Input: dimensioned drawing with shaded views. Units: mm. Origin: part minimum x, y, z. A direction names the side the tool comes from. Round coordinates to 2 decimals unless told otherwise and drop trailing zeros. Order: outer loops, then holes, each group sorted by start corner. A loop starts at its lowest first (then second) coordinate and runs counter-clockwise, first axis right, second up. Notation, with made-up numbers: (42.25, 47.5) - (62.25, 47.5) arc R13 cw to (62.25, 55.5) - close; hole circle Ø11 at (-16.75, 67). An arc over 180 degrees is marked (long way). Put each result on its own line as item: value. Start each with the question number.
(1) Pull-direction query (Y, two-part tool) for the marked faces 4, 5 and 6; classes: released by +Y, released by -Y, zero draft, split by the parting line, or undercut.
(2) Section B-B (x = 36). Output: boundary loops of the cut face in (y, z).
(3) Section D-D (z = 25.5). Output: boundary loops of the cut face in (x, y).
(4) Section C-C (y = 10). Output: boundary loops of the cut face in (x, z).
(5) Material intervals for L1, parallel to X at y = 60.5, z = 17.5; L2, parallel to Y at x = 11, z = 10; L3, parallel to Y at x = 30, z = 16, sorted ascending. Write a range as [from, to].
(6) Pin query (flat end, axial travel): P1, Ø6, axis at y = 64, z = 24, coming from the -X side; P2, Ø8, axis at y = 41, z = 14, coming from the -X side; P3, Ø20.5, axis at x = 13.5, y = 67, coming from the +Z side; P4, Ø1, axis at x = 31.5, y = 64, coming from the -Z side. Return the tip coordinate at first contact, or that it passes through.
(7) Access query for the marked faces 1, 2 and 3. Directions: +Z, -Z, +X, -X, +Y, -Y. A direction counts if a zero-diameter tool reaches every point of the face in a straight line with its end or side. Return the directions, or none.
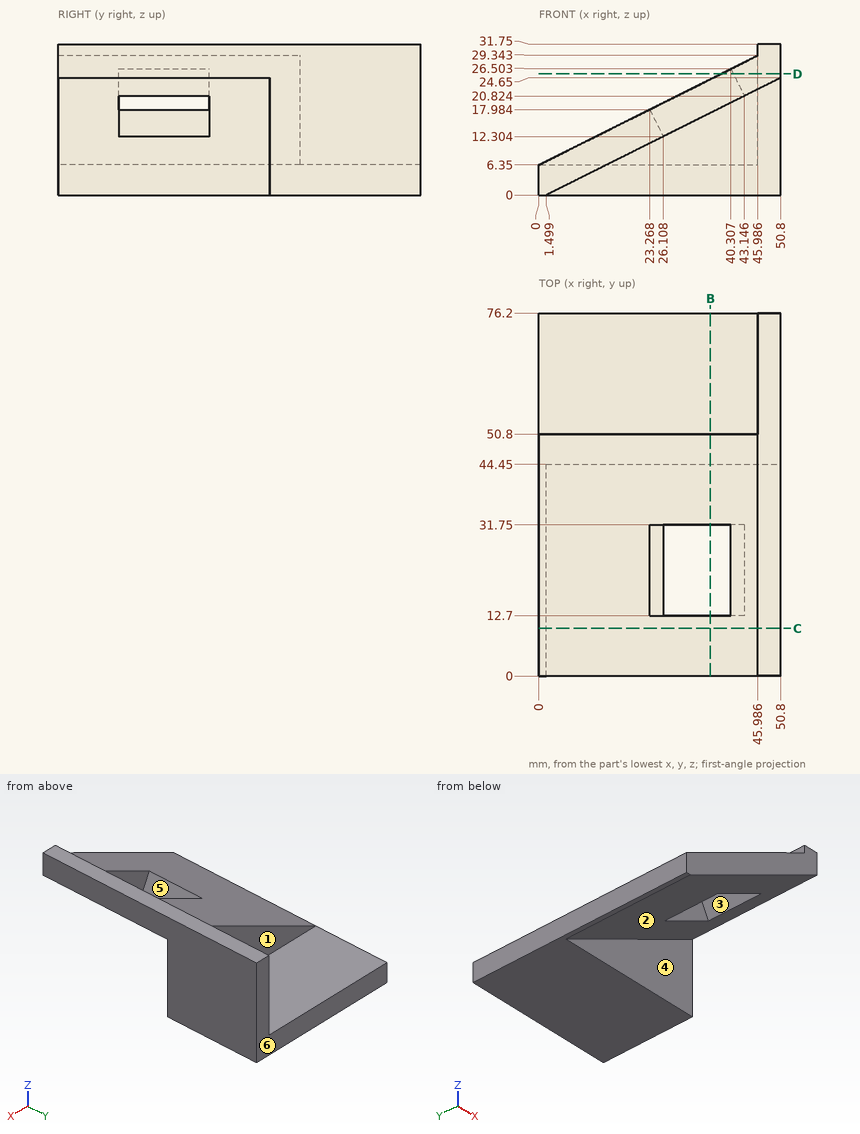
Checks:
1. face 4: released by -Y
1. face 5: undercut
1. face 6: released by +Y
2. outline: (0, 17.25) - (12.7, 17.25) - (12.7, 24.35) - (0, 24.35) - close; (31.75, 17.25) - (44.45, 17.25) - (44.45, 0) - (76.2, 0) - (76.2, 6.35) - (50.8, 6.35) - (50.8, 24.35) - (31.75, 24.35) - close
3. outline: (38.3, 0) - (50.8, 0) - (50.8, 76.2) - (45.99, 76.2) - (45.99, 50.8) - (38.3, 50.8) - (38.3, 31.75) - (40.81, 31.75) - (40.81, 12.7) - (38.3, 12.7) - close
4. outline: (0, 0) - (1.5, 0) - (50.8, 24.65) - (50.8, 31.75) - (45.99, 31.75) - (45.99, 29.34) - (0, 6.35) - close
5. L1: x = [45.99, 50.8]
5. L2: y = [0, 50.8]
5. L3: y = [0, 12.7], [31.75, 50.8]
6. P1: stops at x = 45.99
6. P2: stops at x = 7.3
6. P3: stops at z = 6.35
6. P4: stops at z = 0
7. face 1: +Z, -X, +Y
7. face 2: -Z, +X, -Y
7. face 3: -Z, -X
